from build123d import *

# Parameters (mm, degrees)
SKETCH1_R                    = 1.7
BOSS_EXTRUDE1_DEPTH          = 1.5
BOSS_EXTRUDE2_START          = 1.5
SKETCH1_3_R                  = 1.7
BOSS_EXTRUDE2_DEPTH          = 1.5
FILLET1_R                    = 1
SKETCH2_R                    = 1.7
BOSS_EXTRUDE3_DEPTH          = 5.3
SKETCH3_R                    = 2.6
CUT_EXTRUDE1_DEPTH           = 3.9
CUT_EXTRUDE1_DRAFT           = -1.5
CUT_EXTRUDE1_PROFILE_2_DEPTH = 3.9
CUT_EXTRUDE1_PROFILE_2_DRAFT = -1.5


with BuildPart() as part:
    # Sketch1 → Boss-Extrude1 (new body)
    with BuildSketch(Plane(origin=(-13.45, 0, 0), x_dir=(0, 0, -1), z_dir=(1, 0, 0))):
        with BuildLine():
            ThreePointArc((-36.90383834, 70.970720842), (-34.276657251, 77.531707495), (-30.494426781, 83.501913439))
            Line((-30.494426781, 83.501913439), (-34.143188918, 85.401338783))
            Line((-34.143188918, 85.401338783), (-51.094135774, 78.867013321))
            Line((-51.094135774, 78.867013321), (-57.13269116, 80.48503936))
            Line((-57.13269116, 80.48503936), (-59.720881611, 70.825781097))
            Line((-59.720881611, 70.825781097), (-45.836878975, 67.105573803))
            Line((-45.836878975, 67.105573803), (-36.90383834, 70.970720842))
        make_face()
        with Locations(Location((-52.631231428, 74.102495958, 0), (0, 0, 270))):
            Circle(SKETCH1_R, mode=Mode.SUBTRACT)
        with Locations(Location((-42.971973165, 71.514305507, 0), (0, 0, 270))):
            Circle(SKETCH1_R, mode=Mode.SUBTRACT)
    extrude(amount=BOSS_EXTRUDE1_DEPTH)

    # Sketch1<3> → Boss-Extrude2 (add)
    with BuildSketch(Plane(origin=(-13.45, 0, 0), x_dir=(0, 0, -1), z_dir=(1, 0, 0)).offset(BOSS_EXTRUDE2_START)):
        with BuildLine():
            Line((-34.143188918, 85.401338783), (-51.094135774, 78.867013321))
            Line((-51.094135774, 78.867013321), (-57.13269116, 80.48503936))
            Line((-57.13269116, 80.48503936), (-59.720881611, 70.825781097))
            Line((-59.720881611, 70.825781097), (-45.836878975, 67.105573803))
            Line((-45.836878975, 67.105573803), (-34.166912695, 72.154933529))
            Line((-34.166912695, 72.154933529), (-32.702433972, 71.39257416))
            ThreePointArc((-32.702433972, 71.39257416), (-31.885174228, 71.344912946), (-31.30617274, 71.923654993))
            ThreePointArc((-31.30617274, 71.923654993), (-29.303876098, 76.233694761), (-26.711829723, 80.21702631))
            ThreePointArc((-26.711829723, 80.21702631), (-26.533623916, 81.040191312), (-27.047449161, 81.707530466))
            Line((-27.047449161, 81.707530466), (-34.143188918, 85.401338783))
        make_face()
        with Locations(Location((-52.631231428, 74.102495958, 0), (0, 0, 270))):
            Circle(SKETCH1_3_R, mode=Mode.SUBTRACT)
        with Locations(Location((-42.971973165, 71.514305507, 0), (0, 0, 270))):
            Circle(SKETCH1_3_R, mode=Mode.SUBTRACT)
    extrude(amount=BOSS_EXTRUDE2_DEPTH)

    # Fillet1
    fillet1_edges = [part.edges().sort_by_distance(p)[0] for p in [
        (-11.95, 77.531707495, 34.276657251),
    ]]
    fillet(fillet1_edges, radius=FILLET1_R)

    # Sketch2 → Boss-Extrude3 (add)
    with BuildSketch(Plane(origin=(-10.45, 0, 0), x_dir=(0, 0, -1), z_dir=(1, 0, 0))):
        with BuildLine():
            Line((-34.166912695, 72.154933529), (-36.210992136, 64.526325198))
            Line((-36.210992136, 64.526325198), (-45.836878975, 67.105573803))
            Line((-45.836878975, 67.105573803), (-59.720881611, 70.825781097))
            Line((-59.720881611, 70.825781097), (-57.13269116, 80.48503936))
            Line((-57.13269116, 80.48503936), (-51.094135774, 78.867013321))
            Line((-51.094135774, 78.867013321), (-34.143188918, 85.401338783))
            Line((-34.143188918, 85.401338783), (-27.047449161, 81.707530466))
            ThreePointArc((-27.047449161, 81.707530466), (-26.533623916, 81.040191312), (-26.711829723, 80.21702631))
            ThreePointArc((-26.711829723, 80.21702631), (-29.303876098, 76.233694761), (-31.30617274, 71.923654993))
            ThreePointArc((-31.30617274, 71.923654993), (-31.885174228, 71.344912946), (-32.702433972, 71.39257416))
            Line((-32.702433972, 71.39257416), (-34.166912695, 72.154933529))
        make_face()
        with Locations(Location((-42.971973165, 71.514305507, 0), (0, 0, 270))):
            Circle(SKETCH2_R, mode=Mode.SUBTRACT)
        with Locations(Location((-52.631231428, 74.102495958, 0), (0, 0, 270))):
            Circle(SKETCH2_R, mode=Mode.SUBTRACT)
    extrude(amount=BOSS_EXTRUDE3_DEPTH)


with BuildPart() as cut_extrude1_tool:
    # Sketch3 → Cut-Extrude1 (with draft: the straight prism first)
    with BuildSketch(Plane(origin=(-5.15, 0, 0), x_dir=(0, 0, -1), z_dir=(1, 0, 0))):
        with Locations((-52.631231428, 74.102495958)):
            Circle(SKETCH3_R)
    extrude(amount=-CUT_EXTRUDE1_DEPTH)
    # Cut-Extrude1: the draft: its side faces are tilted about the plane it starts from
    cut_extrude1_sides = [cut_extrude1_tool.faces().sort_by_distance(p)[0] for p in [
        (-7.1, 74.102495958, 55.231231428),
    ]]
    draft(cut_extrude1_sides, Plane(origin=(-5.15, 0, 0), x_dir=(0, 0, -1), z_dir=(1, 0, 0)), CUT_EXTRUDE1_DRAFT)


with BuildPart() as part_1:
    add(part.part)

    # Cut-Extrude1: cut by cut_extrude1_tool
    add(cut_extrude1_tool.part, mode=Mode.SUBTRACT)


with BuildPart() as cut_extrude1_profile_2_tool:
    # Sketch3 → Cut-Extrude1 profile 2 (with draft: the straight prism first)
    with BuildSketch(Plane(origin=(-5.15, 0, 0), x_dir=(0, 0, -1), z_dir=(1, 0, 0))):
        with Locations((-42.971973165, 71.514305507)):
            Circle(SKETCH3_R)
    extrude(amount=-CUT_EXTRUDE1_PROFILE_2_DEPTH)
    # Cut-Extrude1 profile 2: the draft: its side faces are tilted about the plane it starts from
    cut_extrude1_profile_2_sides = [cut_extrude1_profile_2_tool.faces().sort_by_distance(p)[0] for p in [
        (-7.1, 71.514305507, 45.571973165),
    ]]
    draft(cut_extrude1_profile_2_sides, Plane(origin=(-5.15, 0, 0), x_dir=(0, 0, -1), z_dir=(1, 0, 0)), CUT_EXTRUDE1_PROFILE_2_DRAFT)


with BuildPart() as part_2:
    add(part_1.part)

    # Cut-Extrude1 profile 2: cut by cut_extrude1_profile_2_tool
    add(cut_extrude1_profile_2_tool.part, mode=Mode.SUBTRACT)


solid = part_2.part
Could you check a few things on this model? Use its own coordinates, in mm. A direction names the side the tool comes from. Give positions to 0.01 mm unless a question says otherwise; leave off trailing zeros. Loops run counter-clockwise (first coordinate to the right, second up) from the corner with the lowest first, then second, coordinate; pieces in that order, holes last. Notation, with made-up numbers: (-12, 53) -> (47, 53) arc R21 ccw to (47, 81) -> close; hole circle Ø1 at (68.5, 72.25). An arc over 180 degrees is marked (long way). Answer as CSV lines item,"result". Start each with the question number.
(1) We'd pull the mould along Z, two halves only. Please class faces 1 (the flat face through (-8.598, 71.768, 33.424)), 2 (the flat face through (-13.45, 76, 45)), 3 (the flat face through (-9.358, 75.588, 58.445)): released by +Z, released by -Z, zero draft, split by the parting line, or undercut.
(2) If we section it at A-A on x = -11.5: Write out the boundary of the cut face in (y, z), then the cut area to 3 significant figures.
(3) If we section it at C-C on z = 48.5: Write out the boundary of the cut face in (x, y), then the cut area to 4 significant figures.
(4) I'm going to push flat-ended pins straight in: pin 1 Ø2.5 at (y, z) = (73, 53.5) entering from +X; pin 2 Ø3 at (x, z) = (-8.5, 51) entering from +Y; pin 3 Ø1 at (x, z) = (-10, 53.5) entering from -Y. Where does each tip first touch, or does it pass through?
(5) If we section it at B-B on x = -6: Write out the boundary of the cut face in (y, z).
(6) If we section it at D-D on y = 66.25: Write out the boundary of the cut face in (x, z), then the cut area to 3 significant figures.
(7) Which directions (+Z, -Z, +X, -X, +Y, -Y) give clear straight access to the entire face, cutting with the end or side of a thin tool? Please do faces 4 (the conical face through (-7.07, 76.25, 51.26)), 5 (the flat face through (-9.358, 82.088, 42.737)), 6 (the cylindrical face through (-13.204, 77.443, 34.322)).
(8) I need wall thicknesses on probe 1 along X at (y, z) = (72.75, 35); probe 2 along Z at (x, y) = (-12.5, 75) (3 decimals); probe 3 along X at (y, z) = (66.5, 40.5). Which ranges of each line are inside material? Lowest first, please.
Computed:
1,face 1,"undercut"
1,face 2,"zero draft"
1,face 3,"released by +Z"
2,outline,"(67.11, 45.84) -> (72.15, 34.17) -> (71.39, 32.7) arc R1 ccw to (71.92, 31.31) arc R33.5 cw to (80.22, 26.71) arc R1 ccw to (81.71, 27.05) -> (85.4, 34.14) -> (78.87, 51.09) -> (80.49, 57.13) -> (70.83, 59.72) -> close; hole circle Ø3.4 at (71.51, 42.97); hole circle Ø3.4 at (74.1, 52.63)"
2,area,"345 mm2"
3,outline,"(-13.45, 67.82) -> (-5.15, 67.82) -> (-5.15, 79.87) -> (-13.45, 79.87) -> close"
3,area,"100.0 mm2"
4,pin 1,"stops at x = -5.15"
4,pin 2,"stops at y = 79.48"
4,pin 3,"stops at y = 69.02"
5,outline,"(64.53, 36.21) -> (72.15, 34.17) -> (71.39, 32.7) arc R1 ccw to (71.92, 31.31) arc R33.5 cw to (80.22, 26.71) arc R1 ccw to (81.71, 27.05) -> (85.4, 34.14) -> (78.87, 51.09) -> (80.49, 57.13) -> (70.83, 59.72) -> close; hole circle Ø5.16 at (71.51, 42.97); hole circle Ø5.16 at (74.1, 52.63)"
6,outline,"(-10.45, 35.75) -> (-5.15, 35.75) -> (-5.15, 42.64) -> (-10.45, 42.64) -> close"
6,area,"36.5 mm2"
7,face 4,"+X"
7,face 5,"+X, -X, +Y"
7,face 6,"-Z, -X, -Y"
8,probe 1,"x = -11.95 to -5.15"
8,probe 2,"z = 35.342 to 51.187, 54.075 to 58.602"
8,probe 3,"x = -10.45 to -5.15"
